Here's how the part is built. I have some questions about the finished solid (model axes, mm). Face numbers are marked on the shaded views. A direction names the side the tool comes from. Coordinates: 2 decimals unless noted, no trailing zeros. Write each loop counter-clockwise with the first axis right and the second up, starting at its lowest first coordinate (ties: lowest second). Pieces come first, ordered by that corner, then holes. Notation, with made-up numbers: (8.25, 17.5) -> (55.25, 17.5) arc R14 cw to (55.25, 22.5) -> close; hole circle Ø8 at (10.25, 21). An arc over 180 degrees is marked (long way). Use CSV: the item, a comma, the result in double quotes. Start each with the question number.
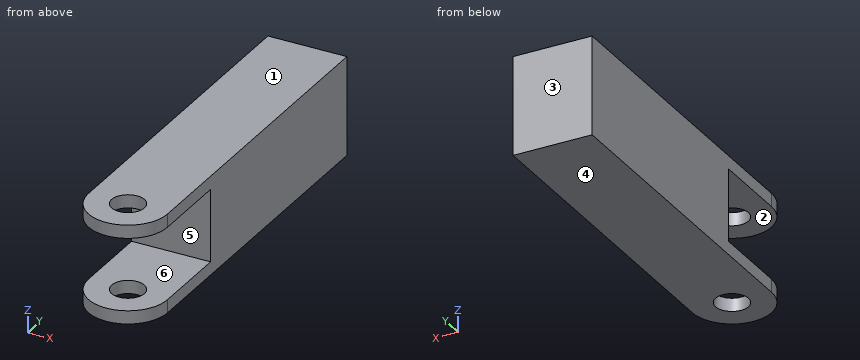
```python
from build123d import *

# Parameters (mm, degrees)
SKETCH1_R               = 2.5
BOSS_EXTRUDE2_DEPTH     = 7.5
CUT_EXTRUDE1_DEPTH      = 51.914143418
CUT_EXTRUDE1_DEPTH_BACK = 51.914143418
SKETCH2_W               = 11
SKETCH2_H               = 34.501138588


with BuildPart() as part:
    # Sketch1 → Boss-Extrude2 (new, symmetric)
    with BuildSketch(Plane.XY):
        with BuildLine():
            Line((-6, 0), (-6, 50))
            Line((-6, 50), (6, 50))
            Line((6, 50), (6, 0))
            ThreePointArc((6, 0), (0, -6), (-6, 0))
        make_face()
        Circle(SKETCH1_R, mode=Mode.SUBTRACT)
    extrude(amount=BOSS_EXTRUDE2_DEPTH, both=True)

    # Sketch2 → Cut-Extrude1 (cut, two sides: drawn at the far end of the back side and taken through both)
    with BuildSketch(Plane(origin=(0, 0, 0), x_dir=(0, 0, -1), z_dir=(1, 0, 0)).offset(-CUT_EXTRUDE1_DEPTH_BACK)):
        with Locations((0, -5.250569294)):
            Rectangle(SKETCH2_W, SKETCH2_H)
    extrude(amount=CUT_EXTRUDE1_DEPTH + CUT_EXTRUDE1_DEPTH_BACK, mode=Mode.SUBTRACT)


solid = part.part
```
Item 1: I want a section at A-A on x = 0. Please give me the cut outline in (y, z).
Item 2: I want a section at D-D on z = 1.5. Please give me the cut outline in (x, y), then the cut area to 3 significant figures.
Item 3: If I drill on line 1 along Y through (x, z) = (0, 6.7); line 2 along X through (y, z) = (0, 6.65); line 3 along Z through (x, y) = (0.75, 7), over which ranges is the centre line in solid material (lowest first)?
Item 4: I'm going to push a flat-ended pin straight in: pin 1 (2 mm diameter, centred on x = -1, z = -5, fed in from -Y). Where does the tip first touch, or does it pass through?
Item 5: Which directions (+Z, -Z, +X, -X, +Y, -Y) give clear straight access to the entire face, cutting with the end or side of a thin tool? Please do the marked faces 1 and 2.
Item 6: Thinking about a two-plate mould opening in Z: for the marked faces 3, 4, 5 and 6, which applies, +Z half, -Z half, draft (parallel to the pull), parting line (faces both ways), or undercut?
Item 7: I want a section at C-C on x = -4.25. Please give me the cut outline in (y, z).
Item 8: I want a section at B-B on z = -6.25. Please give me the cut outline in (x, y).
Geometry says:
1,outline,"(-6, -7.5) -> (-2.5, -7.5) -> (-2.5, -5.5) -> (-6, -5.5) -> close; (-6, 5.5) -> (-2.5, 5.5) -> (-2.5, 7.5) -> (-6, 7.5) -> close; (2.5, -7.5) -> (50, -7.5) -> (50, 7.5) -> (2.5, 7.5) -> (2.5, 5.5) -> (12, 5.5) -> (12, -5.5) -> (2.5, -5.5) -> close"
2,outline,"(-6, 12) -> (6, 12) -> (6, 50) -> (-6, 50) -> close"
2,area,"456 mm2"
3,line 1,"-6 to -2.5, 2.5 to 50"
3,line 2,"-6 to -2.5, 2.5 to 6"
3,line 3,"-7.5 to -5.5, 5.5 to 7.5"
4,pin 1,"y = -6"
5,face 1,"+Z, +X, -X, +Y, -Y"
5,face 2,"+X, -X, -Y"
6,face 3,"draft"
6,face 4,"-Z half"
6,face 5,"undercut"
6,face 6,"undercut"
7,outline,"(-4.24, -7.5) -> (50, -7.5) -> (50, 7.5) -> (-4.24, 7.5) -> (-4.24, 5.5) -> (12, 5.5) -> (12, -5.5) -> (-4.24, -5.5) -> close"
8,outline,"(-6, 0) arc R6 ccw to (6, 0) -> (6, 50) -> (-6, 50) -> close; hole circle Ø5 at (0, 0)"
